Build history of the part. All positions in model axes, mm. Face numbers are marked on the shaded views. A direction names the side the tool comes from. Round coordinates to 2 decimals unless told otherwise and drop trailing zeros. Order: outer loops, then holes, each group sorted by start corner. A loop starts at its lowest first (then second) coordinate and runs counter-clockwise, first axis right, second up. Notation, with made-up numbers: (21.25, 56.25) -> (69.25, 56.25) arc R33 cw to (69.25, 90.25) -> close; hole circle Ø10 at (64.5, 43.5). An arc over 180 degrees is marked (long way). Use a Markdown table: item, result. Add a question column.
Item 1: Probe L1, parallel to X at y = 21.25, z = 0; L2, parallel to Y at x = -5.5, z = 20; L3, parallel to Z at x = -18, y = 23.5. List the from-to ranges inside material, lowest first.
Item 2: Slice it at A-A, the plane x = 0. Give the cut face in (y, z), plus the area to 3 significant figures.
Item 3: Slice it at B-B, the plane z = 0. Give the cut face in (x, y).
Item 4: Two-plate mould, pull along Z, no slides. Class the marked faces 1, 2, 3 and 4: released by +Z, released by -Z, zero draft, split by the parting line, or undercut.
Item 5: 3-axis set-ups, long thin cutter, end or side, ignore diameter. For the marked faces 5 and 6: which of +Z, -Z, +X, -X, +Y, -Y reach the whole face in a straight line?
Item 6: Slice it at D-D, the plane y = 4.5. Give the cut face in (x, z).
Item 7: Slice it at C-C, the plane y = 15.5. Give the cut face in (x, z).
Item 8: Pin check, flat tips, straight feed: pin 1 (6 mm diameter, centred on x = -17.5, z = -24.5, fed in from -Y); pin 2 (2 mm diameter, centred on x = -14, y = 11.5, fed in from +Z); pin 3 (6 mm diameter, centred on x = 9.5, y = 21.5, fed in from +Z); pin 4 (6 mm diameter, centred on x = -2, z = 2.5, fed in from +Y). Stop position of each tip, or through.
from build123d import *

# Parameters (mm, degrees)
SKETCH_1_R          = 32.5
SKETCH_1_R_2        = 5.7
EXTRUDE_1_DEPTH     = 26
SKETCH_2_R          = 25
CUT_EXTRUDE_1_DEPTH = 11.8
FILLET_1_R          = 2


with BuildPart() as part:
    # 草图1 → 凸台-拉伸1 (new body)
    with BuildSketch(Plane(origin=(0, 0, 0), x_dir=(1, 0, 0), z_dir=(0, 1, 0))):
        with Locations(Location((0, 0, 0), (0, 0, 90))):
            Circle(SKETCH_1_R)
        with Locations(Location((0, 0, 0), (0, 0, 90))):
            Circle(SKETCH_1_R_2, mode=Mode.SUBTRACT)
    extrude(amount=EXTRUDE_1_DEPTH)

    # 草图2 → 切除-拉伸1 (cut)
    with BuildSketch(Plane(origin=(0, 26, 0), x_dir=(1, 0, 0), z_dir=(0, 1, 0))):
        with Locations(Location((0, 0, 0), (0, 0, 270))):
            Circle(SKETCH_2_R)
    extrude(amount=-CUT_EXTRUDE_1_DEPTH, mode=Mode.SUBTRACT)

    # 圆角1
    fillet_1_edges = [part.edges().sort_by_distance(p)[0] for p in [
        (0, 0, 32.5),
        (0, 26, 32.5),
    ]]
    fillet(fillet_1_edges, radius=FILLET_1_R)


solid = part.part
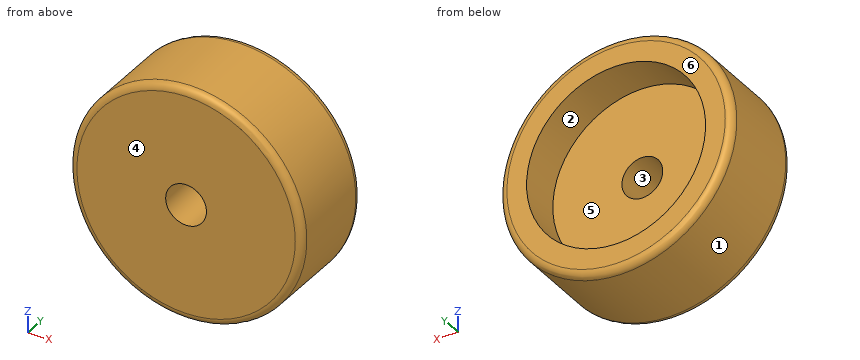
Check sheet entries:
| question | item | result |
|---|---|---|
| 1 | L1 | -32.5 to -25, 25 to 32.5 |
| 1 | L2 | 0 to 14.2 |
| 1 | L3 | -27.06 to -17.35, 17.35 to 27.06 |
| 2 | outline | (0, -30.5) arc R2 ccw to (2, -32.5) -> (24, -32.5) arc R2 ccw to (26, -30.5) -> (26, -25) -> (14.2, -25) -> (14.2, -5.7) -> (0, -5.7) -> close; (0, 5.7) -> (14.2, 5.7) -> (14.2, 25) -> (26, 25) -> (26, 30.5) arc R2 ccw to (24, 32.5) -> (2, 32.5) arc R2 ccw to (0, 30.5) -> close |
| 2 | area | 935 mm2 |
| 3 | outline | (-32.5, 2) arc R2 ccw to (-30.5, 0) -> (-5.7, 0) -> (-5.7, 14.2) -> (-25, 14.2) -> (-25, 26) -> (-30.5, 26) arc R2 ccw to (-32.5, 24) -> close; (5.7, 0) -> (30.5, 0) arc R2 ccw to (32.5, 2) -> (32.5, 24) arc R2 ccw to (30.5, 26) -> (25, 26) -> (25, 14.2) -> (5.7, 14.2) -> close |
| 4 | face 1 | split by the parting line |
| 4 | face 2 | undercut |
| 4 | face 3 | undercut |
| 4 | face 4 | zero draft |
| 5 | face 5 | +Y |
| 5 | face 6 | +Z, -Z, +X, -X, +Y |
| 6 | outline | circle Ø65 at (0, 0); hole circle Ø11.4 at (0, 0) |
| 7 | outline | circle Ø65 at (0, 0); hole circle Ø50 at (0, 0) |
| 8 | pin 1 | y = 0 |
| 8 | pin 2 | z = 29.79 |
| 8 | pin 3 | z = 31.84 |
| 8 | pin 4 | y = 14.2 |
